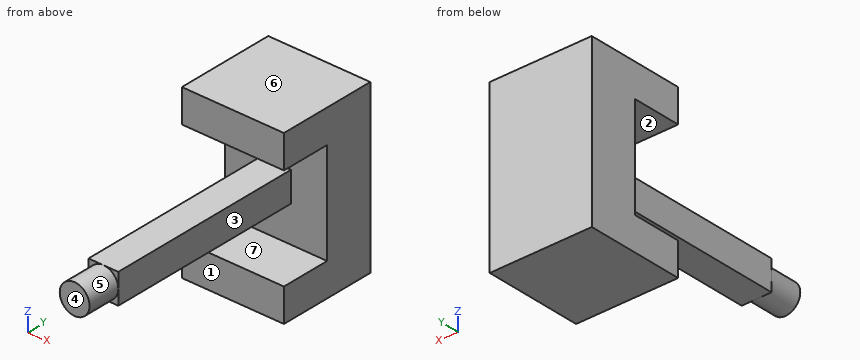
from build123d import *

# Parameters (mm, degrees)
SKETCH1_W           = 1.506666666
SKETCH1_H           = 1.506666666
PIN_DEPTH           = 10
SKETCH2_R           = 0.753333333
TIP_DEPTH           = 1.666666667
SKETCH3_W           = 5.16
SKETCH3_H           = 1.666666667
SKETCH3_H_2         = 5.16
SKETCH3_W_2         = 1.506666666
SKETCH3_H_3         = 1.506666666
HANDLE_DEPTH        = 2.5
SKETCH3_3_W         = 5.16
SKETCH3_3_H         = 1.666666667
BOSS_EXTRUDE4_DEPTH = 2.5


with BuildPart() as part:
    # Sketch1 → Pin (new body)
    with BuildSketch(Plane(origin=(0, 0, 0), x_dir=(1, 0, 0), z_dir=(0, 1, 0))):
        Rectangle(SKETCH1_W, SKETCH1_H)
    extrude(amount=PIN_DEPTH)

    # Sketch2 → Tip (add)
    with BuildSketch(Plane.XZ):
        with Locations(Location((0, 0, 0), (0, 0, 270))):
            Circle(SKETCH2_R)
    extrude(amount=TIP_DEPTH)

    # Sketch3 → Handle (add)
    # profile 1 of 4: a face of its own
    with BuildSketch(Plane(origin=(0, 10, 0), x_dir=(1, 0, 0), z_dir=(0, 1, 0))):
        with Locations((0, 3.413333334)):
            Rectangle(SKETCH3_W, SKETCH3_H)
    # profile 2 of 4: a face of its own
    with BuildSketch(Plane(origin=(0, 10, 0), x_dir=(1, 0, 0), z_dir=(0, 1, 0))):
        Rectangle(SKETCH3_W, SKETCH3_H_2)
        Rectangle(SKETCH3_W_2, SKETCH3_H_3, mode=Mode.SUBTRACT)
    # profile 3 of 4: a face of its own
    with BuildSketch(Plane(origin=(0, 10, 0), x_dir=(1, 0, 0), z_dir=(0, 1, 0))):
        with Locations((0, -3.413333334)):
            Rectangle(SKETCH3_W, SKETCH3_H)
    # profile 4 of 4: a face of its own
    with BuildSketch(Plane(origin=(0, 10, 0), x_dir=(1, 0, 0), z_dir=(0, 1, 0))):
        Rectangle(SKETCH3_W_2, SKETCH3_H_3)
    extrude(amount=HANDLE_DEPTH)

    # Sketch3_3 → Boss-Extrude4 (add)
    with BuildSketch(Plane(origin=(0, 10, 0), x_dir=(1, 0, 0), z_dir=(0, 1, 0))):
        with Locations((0, 3.413333334)):
            Rectangle(SKETCH3_3_W, SKETCH3_3_H)
        with Locations((0, -3.413333334)):
            Rectangle(SKETCH3_3_W, SKETCH3_3_H)
    extrude(amount=-BOSS_EXTRUDE4_DEPTH)


solid = part.part
The model under review builds one solid part; all positions refer to its coordinate system, in mm. Face numbers are marked on the shaded views. A direction names the side the tool comes from. Give positions to 0.01 mm unless a question says otherwise; leave off trailing zeros. Order: outer loops, then holes, each group sorted by start corner. A loop starts at its lowest first (then second) coordinate and runs counter-clockwise, first axis right, second up. Notation, with made-up numbers: M -19.75,85 L -11.75,85 A26 cw -11.75,122 Z; hole C 67,32.5 d9. An arc over 180 degrees is marked long. Use one line per item in the form item = value. Start each with the question number.
Item 1: We need section B-B on x = -1.3. Give the boundary of the cut face in (y, z).
Item 2: The part is to be moulded in two halves that separate along Z. For the marked faces 4, 5, 6 and 7, say which applies: pulls with the +Z half, pulls with the -Z half, needs draft (parallel to the pull), parting line crosses it, or undercut.
Item 3: To check wall thickness, follow line 1 along Z through (x, y) = (0.45, 8.25); line 2 along X through (y, z) = (5, 0.5); line 3 along Y through (x, z) = (-0.6, -3.5). State the ranges of each line that lie inside material, in increasing order. Write a range as from..to.
Item 4: Insertion check: pin 1 Ø0.8 at (x, y) = (0, 3.5) entering from +Z; pin 2 Ø0.8 at (y, z) = (3.5, 0) entering from -X; pin 3 Ø5 at (y, z) = (3.5, -1.5) entering from +X. Each pin has a flat end and moves straight along its axis. Give the tip position at first contact, or say it passes through.
Item 5: We need section C-C on z = -3.25. Give the boundary of the cut face in (x, y), plus the area to 3 significant figures.
Item 6: We need section D-D on y = 0.5. Give the boundary of the cut face in (x, z).
Item 7: For the marked faces 1, 2 and 3, list the 3-axis set-ups (+Z, -Z, +X, -X, +Y, -Y) from which the entire face can be reached by the end or side of a thin tool; tool diameter is ignored.
Item 8: We need section A-A on y = 8. Give the boundary of the cut face in (x, z), plus the area to 3 significant figures.
Completed:
q1.outline = M 7.5,-4.25 L 12.5,-4.25 L 12.5,4.25 L 7.5,4.25 L 7.5,2.58 L 10,2.58 L 10,-2.58 L 7.5,-2.58 Z
q2.face_4 = needs draft
q2.face_5 = parting line crosses it
q2.face_6 = pulls with the +Z half
q2.face_7 = undercut
q3.line_1 = -4.25..-2.58, -0.75..0.75, 2.58..4.25
q3.line_2 = -0.75..0.75
q3.line_3 = 7.5..12.5
q4.pin_1 = 0.75
q4.pin_2 = -0.75
q4.pin_3 = 0.75
q5.outline = M -2.58,7.5 L 2.58,7.5 L 2.58,12.5 L -2.58,12.5 Z
q5.area = 25.8 mm²
q6.outline = M -0.75,-0.75 L 0.75,-0.75 L 0.75,0.75 L -0.75,0.75 Z
q7.face_1 = -Z, +X, -X, -Y
q7.face_2 = +X, -X, -Y
q7.face_3 = +X, -Y
q8.outline = M -2.58,-4.25 L 2.58,-4.25 L 2.58,-2.58 L -2.58,-2.58 Z; M -2.58,2.58 L 2.58,2.58 L 2.58,4.25 L -2.58,4.25 Z; M -0.75,-0.75 L 0.75,-0.75 L 0.75,0.75 L -0.75,0.75 Z
q8.area = 19.5 mm²
